```python
from build123d import *

# Parameters (mm, degrees)
SKETCH1_W           = 101.6
SKETCH1_H           = 57.15
SKETCH1_W_2         = 96.52
SKETCH1_H_2         = 52.07
BOSS_EXTRUDE1_DEPTH = 15.494
SKETCH2_W           = 101.6
SKETCH2_H           = 57.15
SKETCH2_W_2         = 73.025
SKETCH2_H_2         = 28.1178
BOSS_EXTRUDE2_DEPTH = 2.54
SKETCH3_R           = 5
BOSS_EXTRUDE3_DEPTH = 15.494
SKETCH4_R           = 2.415
CUT_EXTRUDE1_DEPTH  = 6.35
SKETCH5_R           = 1.5
CUT_EXTRUDE2_DEPTH  = 7.874
FILLET1_R           = 2.54


with BuildPart() as part:
    # Sketch1 → Boss-Extrude1 (new body)
    with BuildSketch(Plane.XY):
        Rectangle(SKETCH1_W, SKETCH1_H)
        Rectangle(SKETCH1_W_2, SKETCH1_H_2, mode=Mode.SUBTRACT)
    extrude(amount=BOSS_EXTRUDE1_DEPTH)

    # Sketch2 → Boss-Extrude2 (add)
    with BuildSketch(Plane.XY.offset(15.494)):
        Rectangle(SKETCH2_W, SKETCH2_H)
        Rectangle(SKETCH2_W_2, SKETCH2_H_2, mode=Mode.SUBTRACT)
    extrude(amount=BOSS_EXTRUDE2_DEPTH)

    # Sketch3 → Boss-Extrude3 (add)
    with BuildSketch(Plane(origin=(0, 0, 15.494), x_dir=(-1, 0, 0), z_dir=(0, 0, -1))):
        with BuildLine():
            ThreePointArc((-48.26, 19.023454113), (-43.002927797, 18.501467702), (-40.212, 22.987))
            ThreePointArc((-40.212, 22.987), (-40.478199759, 24.59670037), (-41.248454113, 26.035))
            Line((-41.248454113, 26.035), (-48.26, 26.035))
            Line((-48.26, 26.035), (-48.26, 19.023454113))
        make_face()
        with BuildLine():
            Line((-48.26, 26.035), (-41.248454113, 26.035))
            ThreePointArc((-41.248454113, 26.035), (-48.747533906, 26.522533906), (-48.26, 19.023454113))
            Line((-48.26, 19.023454113), (-48.26, 26.035))
        make_face()
        with BuildLine():
            Line((48.26, 26.035), (41.248454113, 26.035))
            ThreePointArc((41.248454113, 26.035), (41.676466094, 19.451466094), (48.26, 19.023454113))
            Line((48.26, 19.023454113), (48.26, 26.035))
        make_face()
        with BuildLine():
            ThreePointArc((50.212, 22.987), (46.82170037, 27.720800241), (41.248454113, 26.035))
            Line((41.248454113, 26.035), (48.26, 26.035))
            Line((48.26, 26.035), (48.26, 19.023454113))
            ThreePointArc((48.26, 19.023454113), (49.697532298, 20.777927797), (50.212, 22.987))
        make_face()
        with BuildLine():
            Line((-48.26, -26.035), (-48.26, -19.023454113))
            ThreePointArc((-48.26, -19.023454113), (-48.747533906, -26.522533906), (-41.248454113, -26.035))
            Line((-41.248454113, -26.035), (-48.26, -26.035))
        make_face()
        with BuildLine():
            ThreePointArc((-40.212, -22.987), (-43.002927797, -18.501467702), (-48.26, -19.023454113))
            Line((-48.26, -19.023454113), (-48.26, -26.035))
            Line((-48.26, -26.035), (-41.248454113, -26.035))
            ThreePointArc((-41.248454113, -26.035), (-40.478199759, -24.59670037), (-40.212, -22.987))
        make_face()
        with Locations((45.212, -22.987)):
            Circle(SKETCH3_R)
    extrude(amount=BOSS_EXTRUDE3_DEPTH)

    # Sketch4 → Cut-Extrude1 (cut)
    with BuildSketch(Plane(origin=(0, 0, 0), x_dir=(-1, 0, 0), z_dir=(0, 0, -1))):
        with Locations((-45.212, 22.987)):
            Circle(SKETCH4_R)
        with Locations((-45.212, -22.987)):
            Circle(SKETCH4_R)
        with Locations((45.212, -22.987)):
            Circle(SKETCH4_R)
        with Locations((45.212, 22.987)):
            Circle(SKETCH4_R)
    extrude(amount=-CUT_EXTRUDE1_DEPTH, mode=Mode.SUBTRACT)

    # Sketch5 → Cut-Extrude2 (cut)
    with BuildSketch(Plane(origin=(0, 0, 6.35), x_dir=(-1, 0, 0), z_dir=(0, 0, -1))):
        with Locations((-45.212, 22.987)):
            Circle(SKETCH5_R)
        with Locations((45.212, -22.987)):
            Circle(SKETCH5_R)
        with Locations((-45.212, -22.987)):
            Circle(SKETCH5_R)
        with Locations((45.212, 22.987)):
            Circle(SKETCH5_R)
    extrude(amount=-CUT_EXTRUDE2_DEPTH, mode=Mode.SUBTRACT)

    # Sketch6 → Cut-Revolve1 (revolve, cut)
    with BuildSketch(Plane(origin=(0, 22.987, 0), x_dir=(0, 0, -1), z_dir=(0, -1, 0)), mode=Mode.PRIVATE) as cut_revolve1_sk:
        Polygon((0, 48.012), (-6.35, 46.892323673), (-6.35, 45.212), (0, 45.212), align=None)
    revolve(cut_revolve1_sk.sketch.rotate(Axis((45.212, 22.987, 6.35), (0, 0, -1)), 180), axis=Axis((45.212, 22.987, 6.35), (0, 0, -1)), mode=Mode.SUBTRACT)

    # Sketch7 → Cut-Revolve2 (revolve, cut)
    with BuildSketch(Plane(origin=(0, -22.987, 0), x_dir=(0, 0, -1), z_dir=(0, 1, 0))):
        Polygon((0, 48.006), (-6.35, 46.886323673), (-6.35, 45.212), (0, 45.212), align=None)
    revolve(axis=Axis((-45.212, -22.987, 6.35), (0, 0, -1)), mode=Mode.SUBTRACT)

    # Sketch8 → Cut-Revolve3 (revolve, cut)
    with BuildSketch(Plane(origin=(0, 22.987, 0), x_dir=(0, 0, -1), z_dir=(0, 1, 0))):
        Polygon((0, 48.006), (-6.35, 46.886323673), (-6.35, 45.212), (0, 45.212), align=None)
    revolve(axis=Axis((-45.212, 22.987, 6.35), (0, 0, -1)), mode=Mode.SUBTRACT)

    # Sketch9 → Cut-Revolve4 (revolve, cut)
    with BuildSketch(Plane(origin=(0, -22.987, 0), x_dir=(0, 0, -1), z_dir=(0, -1, 0)), mode=Mode.PRIVATE) as cut_revolve4_sk:
        Polygon((0, 48.006), (-6.35, 46.886323673), (-6.35, 45.212), (0, 45.212), align=None)
    revolve(cut_revolve4_sk.sketch.rotate(Axis((45.212, -22.987, 6.35), (0, 0, -1)), 180), axis=Axis((45.212, -22.987, 6.35), (0, 0, -1)), mode=Mode.SUBTRACT)

    # Fillet1
    fillet1_edges = [part.edges().sort_by_distance(p)[0] for p in [
        (-50.8, 28.575, 9.017),
        (50.8, 28.575, 9.017),
        (50.8, -28.575, 9.017),
        (-50.8, -28.575, 9.017),
    ]]
    fillet(fillet1_edges, radius=FILLET1_R)


solid = part.part
```
Work out the finished part from the listing and answer in its coordinate system (mm). A direction names the side the tool comes from. Give positions to 0.01 mm unless a question says otherwise; leave off trailing zeros. Loops run counter-clockwise (first coordinate to the right, second up) from the corner with the lowest first, then second, coordinate; pieces in that order, holes last. Notation, with made-up numbers: (62.25, 66.5) -> (69.25, 66.5) arc R3 ccw to (69.25, 70.5) -> close; hole circle Ø7 at (-13, 53). An arc over 180 degrees is marked (long way). Use CSV: the item, a comma, the result in double quotes.
1. The mould has two halves that part along Y. Classify faces 4 (the cylindrical face through (47.128, -24.456, 4.22)), 5 (the flat face through (50.8, 0, 9)), 6 (the flat face through (-1, 28.575, 9)): +Y half, -Y half, draft (parallel to the pull), parting line (faces both ways), or undercut.
Found:
face 4,"undercut"
face 5,"draft"
face 6,"+Y half"
2. The part is cut by section B-B (y = 3.5). Write down the section's boundary in (x, z), then the cut area to 3 significant figures.
Found:
outline,"(-50.8, 0) -> (-48.26, 0) -> (-48.26, 15.49) -> (-36.51, 15.49) -> (-36.51, 18.03) -> (-50.8, 18.03) -> close; (36.51, 15.49) -> (48.26, 15.49) -> (48.26, 0) -> (50.8, 0) -> (50.8, 18.03) -> (36.51, 18.03) -> close"
area,"151 mm^2"
3. Flat-ended cylindrical pins translate along their axes: pin 1 Ø5 at (x, y) = (-8, -21.5) entering from -Z; pin 2 Ø2.5 at (x, y) = (45.212, 22.987) entering from -Z; pin 3 Ø2.5 at (x, y) = (45, 24) entering from -Z. Find the tip coordinate at first contact, or state that the pin passes through.
Found:
pin 1,"z = 15.49"
pin 2,"z = 14.22"
pin 3,"z = 6.35"
4. A tool of negligible diameter and unlimited length cuts with its end or side. For faces 1 (the flat face through (-1, 14.059, 17)), 2 (the flat face through (-45, 23, 14.224)), 3 (the cylindrical face through (-50.076, 27.811, 8.891)), from which of +Z, -Z, +X, -X, +Y, -Y can it reach the whole face along a straight path? Write none if from no direction.
Found:
face 1,"+Z, -Z"
face 2,"-Z"
face 3,"+Z, -Z, -X, +Y"
5. The part is cut by section A-A (z = 5). Write down the section's boundary in (x, y) (3 decimals), then the cut area to 3 significant figures.
Found:
outline,"(-50.8, -26.035) arc R2.54 ccw to (-48.26, -28.575) -> (48.26, -28.575) arc R2.54 ccw to (50.8, -26.035) -> (50.8, 26.035) arc R2.54 ccw to (48.26, 28.575) -> (-48.26, 28.575) arc R2.54 ccw to (-50.8, 26.035) -> close; hole (-48.26, -19.023) arc R5 cw to (-41.248, -26.035) -> (41.248, -26.035) arc R5 cw to (48.26, -19.023) -> (48.26, 19.023) arc R5 cw to (41.248, 26.035) -> (-41.248, 26.035) arc R5 cw to (-48.26, 19.023) -> close; hole circle Ø4.83 at (-45.212, -22.987); hole circle Ø4.83 at (-45.212, 22.987); hole circle Ø4.83 at (45.212, -22.987); hole circle Ø4.83 at (45.212, 22.987)"
area,"931 mm^2"
6. Straight lines are drawn through the part: line 1 (X direction, y = 11.5, z = 5.75); line 2 (Y direction, x = 27, z = 14.5) (3 decimals); line 3 (X direction, y = -24, z = 13.75). For each, find the intervals that lie inside material, in ascending order.
Found:
line 1,"-50.8 to -48.26, 48.26 to 50.8"
line 2,"-28.575 to -26.035, 26.035 to 28.575"
line 3,"-50.8 to -46.32, -44.11 to -40.32, 40.32 to 44.11, 46.32 to 50.8"
7. The part is cut by section D-D (z = 16.5). Write down the section's boundary in (x, y) (1 decimal).
Found:
outline,"(-50.8, -26) arc R2.5 ccw to (-48.3, -28.6) -> (48.3, -28.6) arc R2.5 ccw to (50.8, -26) -> (50.8, 26) arc R2.5 ccw to (48.3, 28.6) -> (-48.3, 28.6) arc R2.5 ccw to (-50.8, 26) -> close; hole (-36.5, -14.1) -> (36.5, -14.1) -> (36.5, 14.1) -> (-36.5, 14.1) -> close"
8. The part is cut by section C-C (x = 26). Write down the section's boundary in (y, z) (3 decimals), then the cut area to 3 significant figures.
Found:
outline,"(-28.575, 0) -> (-26.035, 0) -> (-26.035, 15.494) -> (-14.059, 15.494) -> (-14.059, 18.034) -> (-28.575, 18.034) -> close; (14.059, 15.494) -> (26.035, 15.494) -> (26.035, 0) -> (28.575, 0) -> (28.575, 18.034) -> (14.059, 18.034) -> close"
area,"152 mm^2"
